Could you check a few things on this model? Use its own coordinates, in mm. Face numbers are marked on the shaded views. Coordinates: 2 decimals unless noted, no trailing zeros. Order: outer loops, then holes, each group sorted by start corner. A loop starts at its lowest first (then second) coordinate and runs counter-clockwise, first axis right, second up.
Autodesk Inventor part; units mm, degrees
ref_plane "YZ Plane" through (0, 0, 0) normal (1, 0, 0) x (0, 1, 0)
ref_plane "XZ Plane" through (0, 0, 0) normal (0, 1, 0) x (-1, 0, 0)
ref_plane "XY Plane" through (0, 0, 0) normal (0, 0, 1) x (1, 0, 0)
sketch "Boceto1" plane through (0, 0, 0) normal (0, 1, 0) x (-1, 0, 0)
  line L0 (0, 0) -> (600, 0)
  line L1 (600, 0) -> (600, -600)
  line L2 (600, -600) -> (0, -600)
  line L3 (0, -600) -> (0, 0)
  dimension "d0" = 600
  dimension "d1" = 600
extrude "Extrusión1" add sketch "Boceto1" along normal blind 30
fillet "Empalme1" radius 20 4 edges at (-300, 30, 0) (0, 30, -300) (-300, 30, -600) (-600, 30, -300)
sketch "Boceto2" plane through (0, 30, 0) normal (0, 1, 0) x (1, 0, 0)
  circle A0 centre (-350.7134, 158.3807) radius 25
  circle A1 centre (-459.5461, 158.3807) radius 25
  circle A2 centre (-350.7134, 248.7418) radius 25
  circle A3 centre (-459.5461, 248.7418) radius 25
  arc A4 (-195.2633, 121.4375) -> (-130.7405, 121.4375) centre (-163.0019, 121.4375) ccw
  arc A5 (-110.2556, 305.231) -> (-215.7481, 305.231) centre (-163.0019, 317.1367) ccw
  line L0 (-108.9286, 317.1367) -> (-130.7405, 121.4375)
  line L1 (-195.2633, 121.4375) -> (-217.0751, 317.1367)
  arc A6 (-333.7394, 348.6874) -> (-333.7394, 401.4079) centre (-333.7394, 375.0477) ccw
  line L2 (-333.7394, 348.6874) -> (-472.5261, 348.6874)
  line L3 (-333.7394, 401.4079) -> (-472.5261, 401.4079)
  line L4 (-472.5261, 401.4079) -> (-472.5261, 348.6874)
  arc A7 (-331.4434, 446.537) -> (-331.4434, 499.2575) centre (-331.4434, 472.8973) ccw
  line L5 (-331.4434, 446.537) -> (-470.23, 446.537)
  line L6 (-331.4434, 499.2575) -> (-470.23, 499.2575)
  line L7 (-470.23, 499.2575) -> (-470.23, 446.537)
  circle A8 centre (-163.585, 428.2615) radius 10.0613
  circle A9 centre (-118.3661, 472.3141) radius 10.0613
  circle A10 centre (-162.4187, 517.5331) radius 10.0613
  circle A11 centre (-207.6377, 473.4804) radius 10.0613
  line L8 (-118.2811, 462.2532) -> (-147.5182, 456.7387)
  line L9 (-118.3661, 482.3754) -> (-147.0901, 488.3237)
  line L10 (-152.3603, 517.7711) -> (-147.0901, 488.3237)
  line L11 (-172.48, 517.5331) -> (-178.4251, 488.9079)
  line L12 (-208.7596, 483.4789) -> (-178.4251, 488.9079)
  line L13 (-173.6463, 428.2615) -> (-178.9246, 457.3337)
  line L14 (-208.529, 463.4587) -> (-178.9246, 457.3337)
  line L15 (-153.5449, 427.6096) -> (-147.5182, 456.7387)
  point P0 (0, 0)
  point P1 (-163.0019, 472.8973)
  point P2 (-163.0019, 472.8973)
  point P3 (-163.0019, 472.8973)
  point P4 (-163.0019, 472.8973)
  dimension "d5" = 50
  dimension "d6" = 50
  dimension "d7" = 50
  dimension "d8" = 50
  dimension "d11" = 360
extrude "Extrusión2" add sketch "Boceto2" along normal blind 50 contours A0 | A1 | A2 | A3 | L1 A5 L0 A4 | L2 L4 L3 A6 | L5 L7 L6 A7 | A8 | A8 L13 L14 A11 L12 L11 A10 L10 L9 A9 L8 L15 | A11 | A9 | A10
properties part number "Lamina"
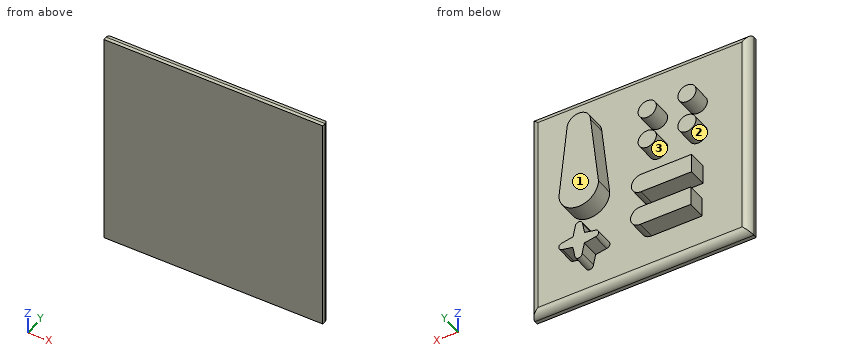
Item 1: Suppose I cut it at B-B (z = -392). List the corners of the cut face in (x, y) for me.
Item 2: Suppose I cut it at C-C (x = -258.5). List the corners of the cut face in (y, z) for me.
Item 3: Suppose I cut it at D-D (z = -101). List the corners of the cut face in (x, y) for me, and give its area (3 significant figures).
Item 4: For pin 1 Ø6 at (x, y) = (-220.5, 27) entering from +Z; pin 2 Ø15 at (x, y) = (-404.5, 64) entering from +Z; pin 3 Ø15 at (y, z) = (60, -387.5) entering from -X; pin 4 Ø10 at (y, z) = (39, -63.5) entering from -X, each with a flat end and sliding along its axis, tell me the tip position at first contact or that it passes through.
Item 5: Thinking about a two-plate mould opening in X: for the marked faces 1, 2 and 3, which applies, +X half, -X half, draft (parallel to the pull), parting line (faces both ways), or undercut?
Item 6: I need wall thicknesses on line 1 (Z direction, x = -384, y = 37); line 2 (X direction, y = 53, z = -228); line 3 (X direction, y = 54, z = -260.5). Which ranges of each line are inside material? Lowest first, please.
Item 7: Suppose I cut it at A-A (y = 69). List the corners of the cut face in (x, z) for me (1 decimal).
Geometry results:
1. outline: (-600, 0) - (0, 0) - (0, 10) arc R20 ccw to (-20, 30) - (-313.55, 30) - (-313.55, 80) - (-472.53, 80) - (-472.53, 30) - (-580, 30) arc R20 ccw to (-600, 10) - close
2. outline: (0, -600) - (10, -600) arc R20 ccw to (30, -580) - (30, -20) arc R20 ccw to (10, 0) - (0, 0) - close
3. outline: (-600, 0) - (0, 0) - (0, 10) arc R20 ccw to (-20, 30) - (-138.04, 30) - (-138.04, 80) - (-187.96, 80) - (-187.96, 30) - (-580, 30) arc R20 ccw to (-600, 10) - close
3. area: 20,300 mm2
4. pin 1: stops at z = -5.72
4. pin 2: stops at z = -348.69
4. pin 3: stops at x = -472.53
4. pin 4: passes through
5. face 1: draft
5. face 2: undercut
5. face 3: undercut
6. line 1: z = -499.26 to -446.54, -401.41 to -348.69
6. line 2: x = -473.5 to -445.59, -364.67 to -336.76, -207.14 to -118.86
6. line 3: x = -481.61 to -437.48, -372.78 to -328.65, -210.76 to -115.24
7. outline: circle Ø50 at (-459.5, -248.7); circle Ø50 at (-459.5, -158.4); (-472.5, -401.4) - (-333.7, -401.4) arc R26.4 ccw to (-333.7, -348.7) - (-472.5, -348.7) - close; (-470.2, -499.3) - (-331.4, -499.3) arc R26.4 ccw to (-331.4, -446.5) - (-470.2, -446.5) - close; circle Ø50 at (-350.7, -248.7); circle Ø50 at (-350.7, -158.4); (-217.1, -317.1) arc R54.1 ccw to (-108.9, -317.1) - (-130.7, -121.4) arc R32.3 ccw to (-195.3, -121.4) - close; (-208.8, -483.5) - (-178.4, -488.9) - (-172.5, -517.5) arc R10.1 ccw to (-152.4, -517.8) - (-147.1, -488.3) - (-118.4, -482.4) arc R10.1 ccw to (-118.3, -462.3) - (-147.5, -456.7) - (-153.5, -427.6) arc R10.1 ccw to (-173.6, -428.3) - (-178.9, -457.3) - (-208.5, -463.5) arc R10.1 ccw to start
